Could you check a few things on this model? Use its own coordinates, in mm. Face numbers are marked on the shaded views. A direction names the side the tool comes from. Coordinates: 2 decimals unless noted, no trailing zeros. Loops run counter-clockwise (first coordinate to the right, second up) from the corner with the lowest first, then second, coordinate; pieces in that order, holes last. Notation, with made-up numbers: M -0.75,25 L 38.25,25 A14 ccw 38.25,49 Z; hole C 75.5,82 d10. An arc over 180 degrees is marked long. Write each question's results on one line, items separated by ' | '.
```python
from build123d import *

# Parameters (mm, degrees)
BOSS_EXTRUDE1_DEPTH = 160
RIB6_REACH          = 143.421
SKETCH4_WALL_W      = 391.884760288
SKETCH4_WALL_H      = 6
CUT_EXTRUDE1_DEPTH  = 198.989898732
SKETCH6_R           = 3
CUT_EXTRUDE2_DEPTH  = 10


with BuildPart() as part:
    # Sketch1 → Boss-Extrude1 (new body)
    with BuildSketch(Plane(origin=(0, 0, 0), x_dir=(1, 0, 0), z_dir=(0, 1, 0))):
        with BuildLine():
            Line((0, 0), (0, 59))
            ThreePointArc((0, 59), (0.292893219, 59.707106781), (1, 60))
            Line((1, 60), (5, 60))
            ThreePointArc((5, 60), (5.707106781, 59.707106781), (6, 59))
            Line((6, 59), (6, 7))
            ThreePointArc((6, 7), (6.292893219, 6.292893219), (7, 6))
            Line((7, 6), (99, 6))
            ThreePointArc((99, 6), (99.707106781, 5.707106781), (100, 5))
            Line((100, 5), (100, 1))
            ThreePointArc((100, 1), (99.707106781, 0.292893219), (99, 0))
            Line((99, 0), (0, 0))
        make_face()
    extrude(amount=BOSS_EXTRUDE1_DEPTH)

    # Sketch4 wall → Rib6 (add, up to next)
    with BuildSketch(Plane(origin=(52.5, 80, -32.5), x_dir=(0.868817459121, 0, 0.495132530467), z_dir=(0.495132530467, 0, -0.868817459121)), mode=Mode.PRIVATE) as rib6_sk1:
        Rectangle(SKETCH4_WALL_W, SKETCH4_WALL_H)
    rib6_tool1 = extrude(rib6_sk1.sketch, amount=-RIB6_REACH, mode=Mode.PRIVATE) - part.part
    add(rib6_tool1.solids().sort_by_distance((52.5, 80, -32.5))[0])

    # Sketch5 → Cut-Extrude1 (cut, through all)
    with BuildSketch(Plane.XY):
        Polygon((100, 160), (50, 160), (100, 130), align=None)
        Polygon((100, 30), (100, 0), (50, 0), align=None)
    extrude(amount=-CUT_EXTRUDE1_DEPTH, mode=Mode.SUBTRACT)

    # Sketch6 → Cut-Extrude2 (cut)
    with BuildSketch(Plane.ZY):
        with Locations((-45, 150)):
            Circle(SKETCH6_R)
        with Locations((-15, 150)):
            Circle(SKETCH6_R)
        with Locations((-15, 10)):
            Circle(SKETCH6_R)
        with Locations((-45, 10)):
            Circle(SKETCH6_R)
    extrude(amount=-CUT_EXTRUDE2_DEPTH, mode=Mode.SUBTRACT)


solid = part.part
```
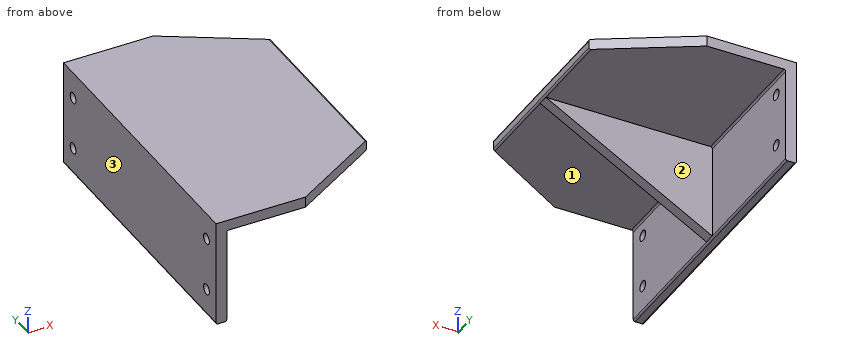
(1) Imagine slicing it at C-C, the plane y = 10. List the corners of the cut face in (x, z) for me.
Reported:
outline: M 0,-59 A1 ccw 1,-60 L 5,-60 A1 ccw 6,-59 L 6,-48 L 0,-48 Z; M 0,-42 L 6,-42 L 6,-18 L 0,-18 Z; M 0,-12 L 6,-12 L 6,-7 A1 cw 7,-6 L 66.67,-6 L 66.67,0 L 0,0 Z
(2) Which directions (+Z, -Z, +X, -X, +Y, -Y) give clear straight access to the entire face, cutting with the end or side of a thin tool? Please do the marked faces 1, 2 and 3.
Reported:
face 1: -Z, +X, -Y | face 2: -Z, +X, +Y | face 3: +Z, -Z, -X, +Y, -Y
(3) Please list where these lines run through material, in increasing order: probe 1 along Y at (x, z) = (4, -45); probe 2 along Z at (x, y) = (3.4, 150); probe 3 along Y at (x, z) = (60.5, -7). Write a range as from..to.
Reported:
probe 1: y = 0..7, 13..147, 153..160 | probe 2: z = -60..-48, -42..-18, -12..0 | probe 3: y = 77..83
(4) Imagine slicing it at A-A, the plane y = 95. List the corners of the cut face in (x, z) for me, and give its area (3 significant figures).
Reported:
outline: M 0,-59 A1 ccw 1,-60 L 5,-60 A1 ccw 6,-59 L 6,-7 A1 cw 7,-6 L 99,-6 A1 ccw 100,-5 L 100,-1 A1 ccw 99,0 L 0,0 Z | area: 923 mm2
(5) Will these pins go through, and if not, where does the flat tip stop? P1, Ø6, axis at x = 17.5, z = -49, coming from the -Y side; P2, Ø3.5, axis at y = 10, z = -15, coming from the -X side; P3, Ø10, axis at y = 92.5, z = -30.5, coming from the +X side; P4, Ø3, axis at x = 64, z = -8, coming from the +Y side.
Reported:
P1: stops at y = 77 | P2: passes through | P3: stops at x = 6 | P4: stops at y = 83
(6) Imagine slicing it at D-D, the plane x = 22. List the corners of the cut face in (y, z) for me.
Reported:
outline: M 0,-6 L 77,-6 L 77,-49.88 L 83,-49.88 L 83,-6 L 160,-6 L 160,0 L 0,0 Z
(7) Imagine slicing it at B-B, the plane z = -15. List the corners of the cut face in (x, y) for me.
Reported:
outline: M 0,0 L 6,0 L 6,7 L 0,7 Z; M 0,13 L 6,13 L 6,77 L 83.21,77 L 83.21,83 L 6,83 L 6,147 L 0,147 Z; M 0,153 L 6,153 L 6,160 L 0,160 Z
